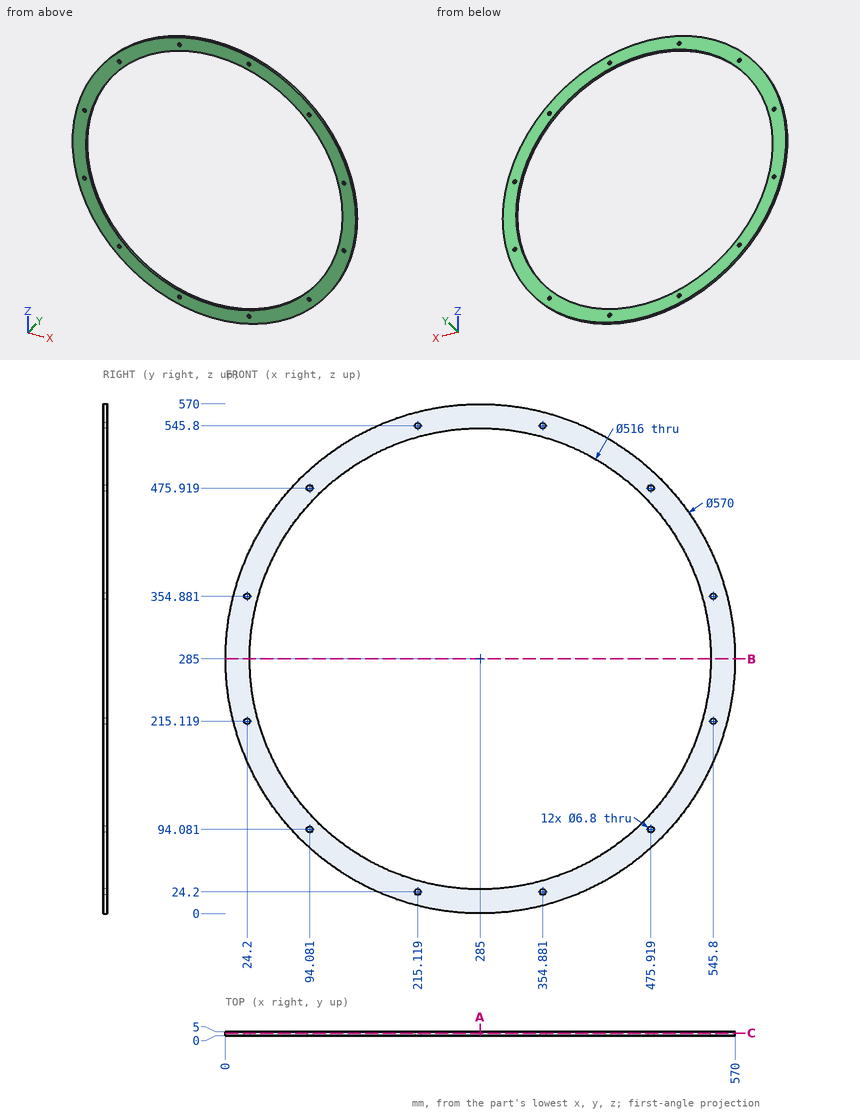
Verification items for this drawing (mm, ordinates from the low corner). Give positions to 0.01 mm unless a question says otherwise; leave off trailing zeros. Write each loop counter-clockwise with the first axis right and the second up, starting at its lowest first coordinate (ties: lowest second). Pieces come first, ordered by that corner, then holes.
1) Section check A-A, the plane x = 285. Record the boundary of the cut face in (y, z).
2) Section check B-B, the plane z = 285. Record the boundary of the cut face in (x, y).
3) Material ranges on L1, parallel to X at y = 4.7, z = 218 (1 decimal); L2, parallel to X at y = 2, z = 291; L3, parallel to X at y = 3.9, z = 289, recorded low to high.
4) Gauge pin test, flat ends, axial feed: pin 1 (2 mm diameter, centred on x = 333.5, y = 2.5, fed in from +Z); pin 2 (1.5 mm diameter, centred on y = 2, z = 82.5, fed in from -X); pin 3 (3 mm diameter, centred on y = 1, z = 139, fed in from -X). Record the tip position at first contact, or that the pin passes through.
5) Section check C-C, the plane y = 3.1. State how many separate pieces and enclosed holes the cut face has, and give its area (3 significant figures).
Computed:
1. outline: (0, 0) - (5, 0) - (5, 27) - (0, 27) - close; (0, 543) - (5, 543) - (5, 570) - (0, 570) - close
2. outline: (0, 0) - (27, 0) - (27, 5) - (0, 5) - close; (543, 0) - (570, 0) - (570, 5) - (543, 5) - close
3. L1: x = 8 to 22.4, 26 to 35.9, 534.1 to 544, 547.6 to 562
3. L2: x = 0.06 to 27.07, 542.93 to 569.94
3. L3: x = 0.03 to 27.03, 542.97 to 569.97
4. pin 1: stops at z = 566.01
4. pin 2: stops at x = 83.7
4. pin 3: stops at x = 39.35
5. separate pieces: 1
5. enclosed holes: 13
5. area: 45,600 mm2
